The figure shows three views and two pictorial views of one solid part (mm, origin at its lowest corner). Answer the questions. Round coordinates to 2 decimals unless told otherwise and drop trailing zeros. Order: outer loops, then holes, each group sorted by start corner. A loop starts at its lowest first (then second) coordinate and runs counter-clockwise, first axis right, second up. Notation, with made-up numbers: (-38, 56) -> (5, 56) arc R26 cw to (5, 85) -> close; hole circle Ø7 at (14.5, -40). An arc over 180 degrees is marked (long way). One line per item, written item: value. Start each with the question number.
1. Consider line 1 (Y direction, x = 54.8, z = 2.5); line 2 (X direction, y = 34.5, z = 3.05); line 3 (Y direction, x = 35, z = 0.6). Determine where each line is inside the solid, lowest interval first.
2. Section B-B (y = 77) is taken. Give the vertices of the cut face in (x, z).
3. Section A-A (x = 3.5) is taken. Give the vertices of the cut face in (y, z).
4. Section D-D (y = 39) is taken. Give the vertices of the cut face in (x, z).
5. Section C-C (x = 15) is taken. Give the vertices of the cut face in (y, z).
6. Flat-ended cylindrical pins translate along their axes: pin 1 Ø2.5 at (y, z) = (47, 1.5) entering from -X; pin 2 Ø2 at (y, z) = (15, 2.5) entering from +X; pin 3 Ø2 at (y, z) = (90, 2.5) entering from -X. Find the tip coordinate at first contact, or state that the pin passes through.
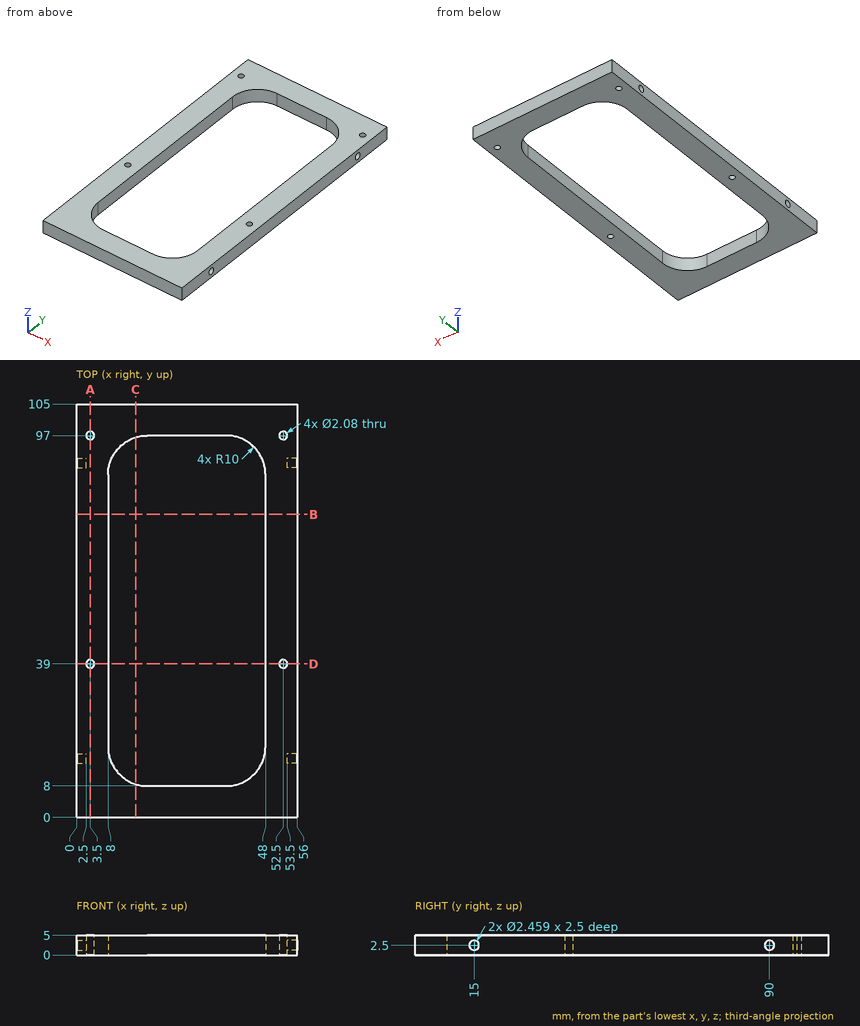
Answer:
1. line 1: 0 to 13.77, 16.23 to 88.77, 91.23 to 105
1. line 2: 0 to 8, 48 to 56
1. line 3: 0 to 8, 97 to 105
2. outline: (0, 0) -> (8, 0) -> (8, 5) -> (0, 5) -> close; (48, 0) -> (56, 0) -> (56, 5) -> (48, 5) -> close
3. outline: (0, 0) -> (37.96, 0) -> (37.96, 5) -> (0, 5) -> close; (40.04, 0) -> (95.96, 0) -> (95.96, 5) -> (40.04, 5) -> close; (98.04, 0) -> (105, 0) -> (105, 5) -> (98.04, 5) -> close
4. outline: (0, 0) -> (2.46, 0) -> (2.46, 5) -> (0, 5) -> close; (4.54, 0) -> (8, 0) -> (8, 5) -> (4.54, 5) -> close; (48, 0) -> (51.46, 0) -> (51.46, 5) -> (48, 5) -> close; (53.54, 0) -> (56, 0) -> (56, 5) -> (53.54, 5) -> close
5. outline: (0, 0) -> (8.46, 0) -> (8.46, 5) -> (0, 5) -> close; (96.54, 0) -> (105, 0) -> (105, 5) -> (96.54, 5) -> close
6. pin 1: x = 0
6. pin 2: x = 53.5
6. pin 3: x = 2.5
